Check sheet for the modelled part. Datum: model origin and axes. Units: mm. Face numbers are marked on the shaded views. A direction names the side the tool comes from. Coordinates: 2 decimals unless noted, no trailing zeros. Loops run counter-clockwise (first coordinate to the right, second up) from the corner with the lowest first, then second, coordinate; pieces in that order, holes last. Notation, with made-up numbers: M 70.25,26 L 81.25,26 A21 cw 81.25,60 Z; hole C 56,25.5 d2. An arc over 180 degrees is marked long. Use CSV: the item, a comma, the result in double quotes. Start each with the question number.
(1) Section check C-C on z = -5.5. Record the cut outline in (x, y), and give its area (3 significant figures).
(2) Section check A-A on x = 0. Record the cut outline in (y, z), and give its area (3 significant figures).
(3) Go/stop test with flat-tipped pins: pin 1 Ø10 at (x, y) = (-3.5, -6) entering from -Z; pin 2 Ø10 at (y, z) = (-3.5, 46) entering from -X; pin 3 Ø2.5 at (y, z) = (-2, -44.5) entering from -X. Record where each tip stops, or that it passes through.
(4) Section check B-B on y = 1.75. Record the cut outline in (x, z), and give its area (3 significant figures).
(5) Section check D-D on y = -6. Record the cut outline in (x, z), and give its area (3 significant figures).
(6) Set-up check for the marked faces 5, 6, 7, 8 and 9: record each of +Z, -Z, +X, -X, +Y, -Y from which the full face is reachable in a straight line by a thin tool's end or side.
(7) Scan lines: line 1 (Z direction, x = 0, y = -8); line 2 (Z direction, x = 35.5, y = -3.25); line 3 (Z direction, x = -3.5, y = 4.75). Record each from-to range of solid material in increasing order.
(8) Draft check along X on the marked faces 1, 2, 3 and 4. Enter one of: pulls with the +X half, pulls with the -X half, needs draft (parallel to the pull), parting line crosses it, or undercut.
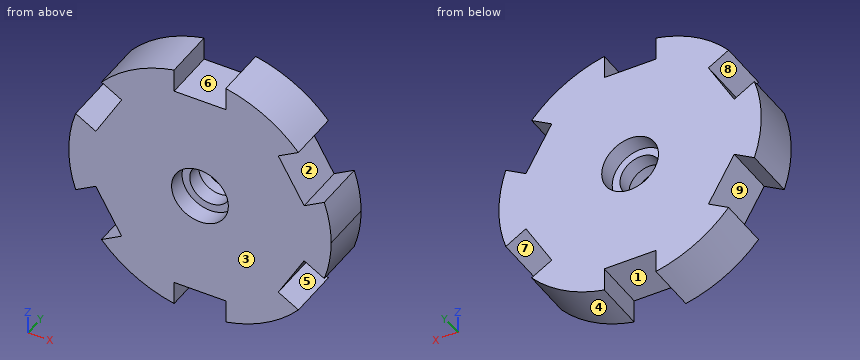
from build123d import *

# Parameters (mm, degrees)
F0_R     = 11
F2_DEPTH = 10.033
F1_R     = 11
F1_R_2   = 8
F3_DEPTH = 3


with BuildPart() as f2:
    # F0 (on Front) → F2 (new body, symmetric)
    with BuildSketch(Plane.XZ):
        with BuildLine():
            ThreePointArc((48.133282, -16.242758), (50.128887, -8.230106), (50.8, 0))
            ThreePointArc((50.8, 0), (50.128887, 8.230106), (48.133282, 16.242758))
            Line((48.133282, 16.242758), (40.333836, 11.739746))
            Line((40.333836, 11.739746), (30.333836, 29.060254))
            Line((30.333836, 29.060254), (38.133282, 33.563266))
            ThreePointArc((38.133282, 33.563266), (25.4, 43.994091), (10, 49.806024))
            Line((10, 49.806024), (10, 40.8))
            Line((10, 40.8), (-10, 40.8))
            Line((-10, 40.8), (-10, 49.806024))
            ThreePointArc((-10, 49.806024), (-25.4, 43.994091), (-38.133282, 33.563266))
            Line((-38.133282, 33.563266), (-30.333836, 29.060254))
            Line((-30.333836, 29.060254), (-40.333836, 11.739746))
            Line((-40.333836, 11.739746), (-48.133282, 16.242758))
            ThreePointArc((-48.133282, 16.242758), (-50.8, 0), (-48.133282, -16.242758))
            Line((-48.133282, -16.242758), (-40.333836, -11.739746))
            Line((-40.333836, -11.739746), (-30.333836, -29.060254))
            Line((-30.333836, -29.060254), (-38.133282, -33.563266))
            ThreePointArc((-38.133282, -33.563266), (-25.4, -43.994091), (-10, -49.806024))
            Line((-10, -49.806024), (-10, -40.8))
            Line((-10, -40.8), (10, -40.8))
            Line((10, -40.8), (10, -49.806024))
            ThreePointArc((10, -49.806024), (25.4, -43.994091), (38.133282, -33.563266))
            Line((38.133282, -33.563266), (30.333836, -29.060254))
            Line((30.333836, -29.060254), (40.333836, -11.739746))
            Line((40.333836, -11.739746), (48.133282, -16.242758))
        make_face()
        Circle(F0_R, mode=Mode.SUBTRACT)
    extrude(amount=F2_DEPTH, both=True)

    # F1 (on Front) → F3 (join, symmetric)
    with BuildSketch(Plane.XZ):
        Circle(F1_R)
        Circle(F1_R_2, mode=Mode.SUBTRACT)
    extrude(amount=F3_DEPTH, both=True)


solid = f2.part
Outcome:
1,outline,"M -50.5,-10.03 L -9.53,-10.03 L -9.53,-3 L -5.81,-3 L -5.81,3 L -9.53,3 L -9.53,10.03 L -50.5,10.03 Z; M 5.81,-3 L 9.53,-3 L 9.53,-10.03 L 50.5,-10.03 L 50.5,10.03 L 9.53,10.03 L 9.53,3 L 5.81,3 Z"
1,area,"1,690 mm²"
2,outline,"M -10.03,-40.8 L 10.03,-40.8 L 10.03,-11 L 3,-11 L 3,-8 L -3,-8 L -3,-11 L -10.03,-11 Z; M -10.03,11 L -3,11 L -3,8 L 3,8 L 3,11 L 10.03,11 L 10.03,40.8 L -10.03,40.8 Z"
2,area,"1,230 mm²"
3,pin 1,"stops at z = -40.8"
3,pin 2,"stops at x = -29.99"
3,pin 3,"stops at x = -26.65"
4,outline,"M -48.13,-16.24 L -40.33,-11.74 L -30.33,-29.06 L -38.13,-33.56 A50.8 ccw -10,-49.81 L -10,-40.8 L 10,-40.8 L 10,-49.81 A50.8 ccw 38.13,-33.56 L 30.33,-29.06 L 40.33,-11.74 L 48.13,-16.24 A50.8 ccw 50.8,0 A50.8 ccw 48.13,16.24 L 40.33,11.74 L 30.33,29.06 L 38.13,33.56 A50.8 ccw 10,49.81 L 10,40.8 L -10,40.8 L -10,49.81 A50.8 ccw -38.13,33.56 L -30.33,29.06 L -40.33,11.74 L -48.13,16.24 A50.8 ccw Z; hole C 0,0 d16"
4,area,"6,750 mm²"
5,outline,"M -48.13,-16.24 L -40.33,-11.74 L -30.33,-29.06 L -38.13,-33.56 A50.8 ccw -10,-49.81 L -10,-40.8 L 10,-40.8 L 10,-49.81 A50.8 ccw 38.13,-33.56 L 30.33,-29.06 L 40.33,-11.74 L 48.13,-16.24 A50.8 ccw 50.8,0 A50.8 ccw 48.13,16.24 L 40.33,11.74 L 30.33,29.06 L 38.13,33.56 A50.8 ccw 10,49.81 L 10,40.8 L -10,40.8 L -10,49.81 A50.8 ccw -38.13,33.56 L -30.33,29.06 L -40.33,11.74 L -48.13,16.24 A50.8 ccw Z; hole C 0,0 d22"
5,area,"6,570 mm²"
6,face 5,"+X, +Y, -Y"
6,face 6,"+Z, +Y, -Y"
6,face 7,"-Z, +Y, -Y"
6,face 8,"-X, +Y, -Y"
6,face 9,"+Y, -Y"
7,line 1,"z = -40.8 to -11, 11 to 40.8"
7,line 2,"z = -36.34 to -32.04, -20.11 to 20.11, 32.04 to 36.34"
7,line 3,"z = -40.8 to -10.43, 10.43 to 40.8"
8,face 1,"undercut"
8,face 2,"undercut"
8,face 3,"needs draft"
8,face 4,"pulls with the +X half"
